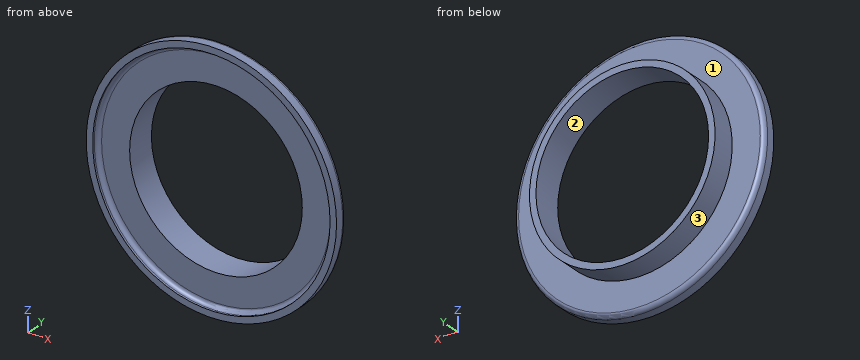
from build123d import *

# Parameters (mm, degrees)
SKETCH1_R                = 21.5
SKETCH1_R_2              = 20
BOSS_EXTRUDE1_DEPTH      = 10
CUT_EXTRUDE1_DEPTH       = 24
CUT_EXTRUDE1_DEPTH_BACK  = 27
SKETCH3_W                = 51.96152563
SKETCH3_H                = 7.978608452
BOSS_EXTRUDE2_DEPTH      = 1.5
BOSS_EXTRUDE2_DEPTH_BACK = 1.5
SKETCH4_R                = 29
SKETCH4_R_2              = 20
SKETCH6_R                = 27.5
CUT_EXTRUDE2_DEPTH       = 1.5
FILLET1_R                = 1


with BuildPart() as part:
    # Sketch1 → Boss-Extrude1 (new body)
    with BuildSketch(Plane(origin=(0, 0, 0), x_dir=(1, 0, 0), z_dir=(0, 1, 0))):
        with Locations(Location((0, 0, 0), (0, 0, 270))):
            Circle(SKETCH1_R)
        with Locations(Location((0, 0, 0), (0, 0, 270))):
            Circle(SKETCH1_R_2, mode=Mode.SUBTRACT)
    extrude(amount=BOSS_EXTRUDE1_DEPTH)

    # Sketch3 → Cut-Extrude1 (cut, two sides: drawn at the far end of the back side and taken through both)
    with BuildSketch(Plane.XY.offset(-CUT_EXTRUDE1_DEPTH_BACK)):
        with Locations((-1.240371902, -1.089304226)):
            Rectangle(SKETCH3_W, SKETCH3_H)
    extrude(amount=CUT_EXTRUDE1_DEPTH + CUT_EXTRUDE1_DEPTH_BACK, mode=Mode.SUBTRACT)

    # Sketch4 → Boss-Extrude2 (add, two sides: drawn at the far end of the back side and taken through both)
    with BuildSketch(Plane.XZ.offset(-2.9).offset(-BOSS_EXTRUDE2_DEPTH_BACK)):
        Circle(SKETCH4_R)
        Circle(SKETCH4_R_2, mode=Mode.SUBTRACT)
    extrude(amount=BOSS_EXTRUDE2_DEPTH + BOSS_EXTRUDE2_DEPTH_BACK)

    # Sketch6 → Cut-Extrude2 (cut)
    with BuildSketch(Plane.XZ.offset(-1.4)):
        Circle(SKETCH6_R)
    extrude(amount=-CUT_EXTRUDE2_DEPTH, mode=Mode.SUBTRACT)

    # Fillet1
    fillet1_edges = [part.edges().sort_by_distance(p)[0] for p in [
        (-29, 4.4, 0),
        (-27.5, 2.9, 0),
    ]]
    fillet(fillet1_edges, radius=FILLET1_R)


solid = part.part
The model under review builds one solid part; all positions refer to its coordinate system, in mm. Face numbers are marked on the shaded views. Give positions to 0.01 mm unless a question says otherwise; leave off trailing zeros. Order: outer loops, then holes, each group sorted by start corner. A loop starts at its lowest first (then second) coordinate and runs counter-clockwise, first axis right, second up. Notation, with made-up numbers: (8.5, -30) -> (36.5, -30) arc R38 cw to (36.5, 9) -> close; hole circle Ø11 at (10.25, 11.5). An arc over 180 degrees is marked (long way). Write item = value, one per line. Start each with the question number.
(1) For pin 1 Ø10 at (x, z) = (-17.5, 0) entering from -Y; pin 2 Ø1 at (y, z) = (4.5, -6.5) entering from +X; pin 3 Ø4 at (x, y) = (-4.5, 2.5) entering from -Z, all flat-tipped, find the tip position at first contact; note any pin that passes through.
(2) Take a section at A-A (x = 0). Write out the cut boundary in (y, z).
(3) Draft analysis for pull direction Z (two halves, no side actions). For the marked faces 1, 2 and 3, state which applies: +Z half, -Z half, draft (parallel to the pull), parting line (faces both ways), or undercut.
(4) For L1, parallel to X at y = 6.25, z = 0; L2, parallel to Z at x = 0, y = 1.65; L3, parallel to X at y = 9, z = 2.5, list the stretches that pass through material, from the lowest coordinate up. Write a range as from..to.
(5) Take a section at C-C (y = 7.5). Write out the cut boundary in (x, z).
(6) Take a section at B-B (z = 0). Write out the cut boundary in (x, y), plus the area to 3 significant figures.
Returned:
q1.pin_1 = 2.9
q1.pin_2 = 28.07
q1.pin_3 = -28.89
q2.outline = (1.4, -29) -> (3.4, -29) arc R1 ccw to (4.4, -28) -> (4.4, -21.5) -> (10, -21.5) -> (10, -20) -> (2.9, -20) -> (2.9, -26.5) arc R1 cw to (1.9, -27.5) -> (1.4, -27.5) -> close; (1.4, 27.5) -> (1.9, 27.5) arc R1 cw to (2.9, 26.5) -> (2.9, 20) -> (10, 20) -> (10, 21.5) -> (4.4, 21.5) -> (4.4, 28) arc R1 ccw to (3.4, 29) -> (1.4, 29) -> close
q3.face_1 = draft
q3.face_2 = undercut
q3.face_3 = parting line
q4.L1 = -21.5..-20, 20..21.5
q4.L2 = -29..-27.5, 27.5..29
q4.L3 = -21.35..-19.84, 19.84..21.35
q5.outline = circle Ø43 at (0, 0); hole circle Ø40 at (0, 0)
q6.outline = (-29, 1.4) -> (-27.5, 1.4) -> (-27.5, 1.9) arc R1 cw to (-26.5, 2.9) -> (-20, 2.9) -> (-20, 10) -> (-21.5, 10) -> (-21.5, 4.4) -> (-28, 4.4) arc R1 ccw to (-29, 3.4) -> close; (20, 2.9) -> (26.5, 2.9) arc R1 cw to (27.5, 1.9) -> (27.5, 1.4) -> (29, 1.4) -> (29, 3.4) arc R1 ccw to (28, 4.4) -> (21.5, 4.4) -> (21.5, 10) -> (20, 10) -> close
q6.area = 48.3 mm²
